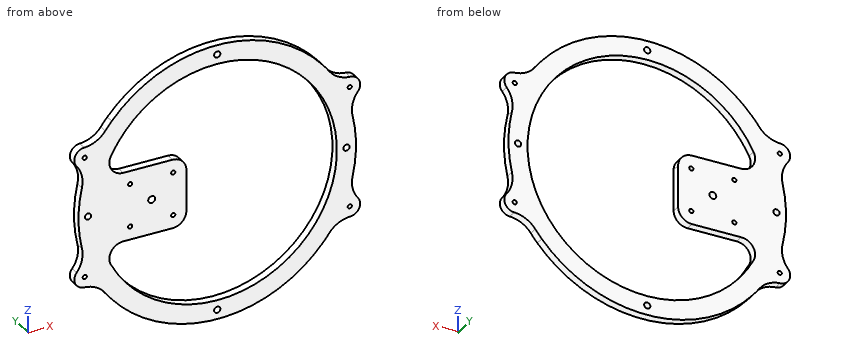
```python
from build123d import *

# Parameters (mm, degrees)
SKETCH1_R           = 86.25
BOSS_EXTRUDE1_DEPTH = 6
SKETCH2_R           = 1.5
CUT_EXTRUDE1_DEPTH  = 6
SKETCH3_R           = 2.25
CUT_EXTRUDE2_DEPTH  = 6
CUT_EXTRUDE3_DEPTH  = 6
FILLET1_R           = 20
SKETCH5_R           = 2.5
SKETCH5_R_2         = 1.5
BOSS_EXTRUDE2_DEPTH = 6
FILLET2_R           = 10


with BuildPart() as part:
    # Sketch1 → Boss-Extrude1 (new body)
    with BuildSketch(Plane(origin=(0, 0, 0), x_dir=(1, 0, 0), z_dir=(0, 1, 0))):
        with BuildLine():
            Line((75.993420768, 65), (110, 65))
            Line((110, 65), (110, -65))
            Line((110, -65), (75.993420768, -65))
            ThreePointArc((75.993420768, -65), (0, -100), (-75.993420768, -65))
            Line((-75.993420768, -65), (-110, -65))
            Line((-110, -65), (-110, 65))
            Line((-110, 65), (-75.993420768, 65))
            ThreePointArc((-75.993420768, 65), (0, 100), (75.993420768, 65))
        make_face()
        Circle(SKETCH1_R, mode=Mode.SUBTRACT)
    extrude(amount=BOSS_EXTRUDE1_DEPTH)

    # Sketch2 → Cut-Extrude1 (cut)
    with BuildSketch(Plane(origin=(0, 0, 0), x_dir=(1, 0, 0), z_dir=(0, 1, 0))):
        with Locations((-95.5, 43.5)):
            Circle(SKETCH2_R)
        with Locations((95.5, 43.5)):
            Circle(SKETCH2_R)
        with Locations((95.5, -43.5)):
            Circle(SKETCH2_R)
        with Locations((-95.5, -43.5)):
            Circle(SKETCH2_R)
    extrude(amount=CUT_EXTRUDE1_DEPTH, mode=Mode.SUBTRACT)

    # Sketch3 → Cut-Extrude2 (cut)
    with BuildSketch(Plane(origin=(0, 0, 0), x_dir=(1, 0, 0), z_dir=(0, 1, 0))):
        with Locations((0, 93.125)):
            Circle(SKETCH3_R)
        with Locations((93.125, 0)):
            Circle(SKETCH3_R)
        with Locations((0, -93.125)):
            Circle(SKETCH3_R)
        with Locations((-93.125, 0)):
            Circle(SKETCH3_R)
    extrude(amount=CUT_EXTRUDE2_DEPTH, mode=Mode.SUBTRACT)

    # Sketch4 → Cut-Extrude3 (cut)
    with BuildSketch(Plane(origin=(0, 0, 0), x_dir=(1, 0, 0), z_dir=(0, 1, 0))):
        with BuildLine():
            Line((98.608905775, -36.674701114), (93.856581268, -34.510029742))
            ThreePointArc((93.856581268, -34.510029742), (100, 0), (93.856581268, 34.510029742))
            Line((93.856581268, 34.510029742), (98.608905775, 36.674701114))
            ThreePointArc((98.608905775, 36.674701114), (102.325298886, 46.608905775), (92.391094225, 50.325298886))
            Line((92.391094225, 50.325298886), (87.638769717, 48.160627513))
            ThreePointArc((87.638769717, 48.160627513), (82.248188777, 56.879130117), (75.993420768, 65))
            Line((75.993420768, 65), (110, 65))
            Line((110, 65), (110, -65))
            Line((110, -65), (75.993420768, -65))
            ThreePointArc((75.993420768, -65), (82.248188777, -56.879130117), (87.638769717, -48.160627513))
            Line((87.638769717, -48.160627513), (92.391094225, -50.325298886))
            ThreePointArc((92.391094225, -50.325298886), (102.325298886, -46.608905775), (98.608905775, -36.674701114))
        make_face()
        with BuildLine():
            Line((-98.608905775, 36.674701114), (-93.856581268, 34.510029742))
            ThreePointArc((-93.856581268, 34.510029742), (-100, 0), (-93.856581268, -34.510029742))
            Line((-93.856581268, -34.510029742), (-98.608905775, -36.674701114))
            ThreePointArc((-98.608905775, -36.674701114), (-102.325298886, -46.608905775), (-92.391094225, -50.325298886))
            Line((-92.391094225, -50.325298886), (-87.638769717, -48.160627513))
            ThreePointArc((-87.638769717, -48.160627513), (-82.248188777, -56.879130117), (-75.993420768, -65))
            Line((-75.993420768, -65), (-110, -65))
            Line((-110, -65), (-110, 65))
            Line((-110, 65), (-75.993420768, 65))
            ThreePointArc((-75.993420768, 65), (-82.248188777, 56.879130117), (-87.638769717, 48.160627513))
            Line((-87.638769717, 48.160627513), (-92.391094225, 50.325298886))
            ThreePointArc((-92.391094225, 50.325298886), (-102.325298886, 46.608905775), (-98.608905775, 36.674701114))
        make_face()
    extrude(amount=CUT_EXTRUDE3_DEPTH, mode=Mode.SUBTRACT)

    # Fillet1
    fillet1_edges = [part.edges().sort_by_distance(p)[0] for p in [
        (87.638769717, 3, -48.160627513),
        (93.856581268, 3, -34.510029742),
        (93.856581268, 3, 34.510029742),
        (87.638769717, 3, 48.160627513),
        (-87.638769717, 3, 48.160627513),
        (-93.856581268, 3, 34.510029742),
        (-93.856581268, 3, -34.510029742),
        (-87.638769717, 3, -48.160627513),
    ]]
    fillet(fillet1_edges, radius=FILLET1_R)

    # Sketch5 → Boss-Extrude2 (add)
    with BuildSketch(Plane(origin=(0, 0, 0), x_dir=(1, 0, 0), z_dir=(0, 1, 0))):
        Polygon((-72.25, 25), (-22.25, 25), (-22.25, -25), (-72.25, -25), (-87.689436508, -25), (-87.689436508, 25), align=None)
        with Locations((-47.25, 0)):
            Circle(SKETCH5_R, mode=Mode.SUBTRACT)
        with Locations((-62.75, 15.5)):
            Circle(SKETCH5_R_2, mode=Mode.SUBTRACT)
        with Locations((-31.75, 15.5)):
            Circle(SKETCH5_R_2, mode=Mode.SUBTRACT)
        with Locations((-62.75, -15.5)):
            Circle(SKETCH5_R_2, mode=Mode.SUBTRACT)
        with Locations((-31.75, -15.5)):
            Circle(SKETCH5_R_2, mode=Mode.SUBTRACT)
    extrude(amount=BOSS_EXTRUDE2_DEPTH)

    # Fillet2
    fillet2_edges = [part.edges().sort_by_distance(p)[0] for p in [
        (-82.547334905, 3, 25),
        (-82.547334905, 3, -25),
        (-22.25, 3, 25),
        (-22.25, 3, -25),
    ]]
    fillet(fillet2_edges, radius=FILLET2_R)


solid = part.part
```
Can you work these out from the model? Positions are in its coordinate system, mm. Round coordinates to 2 decimals unless told otherwise and drop trailing zeros. Loops run counter-clockwise (first coordinate to the right, second up) from the corner with the lowest first, then second, coordinate; pieces in that order, holes last. Notation, with made-up numbers: M 21.5,63.5 L 61.5,63.5 A21 cw 61.5,92.5 Z; hole C 63,38 d8. An arc over 180 degrees is marked long. Answer as a JSON object with one key per item and string values. Group by question number.
Q1. Please list where these lines run through material, in increasing order: L1, parallel to Z at x = -95.5, y = 4.4; L2, parallel to Z at x = -47.25, y = 3.9; L3, parallel to Z at x = -54.5, y = 1.5.
Q2. Will these pins go through, and if not, where does the flat tip stop? pin 1 (3 mm diameter, centred on x = -41.5, y = 2.5, fed in from -Z); pin 2 (1.8 mm diameter, centred on x = -31.75, z = 15.5, fed in from +Y); pin 3 (1.5 mm diameter, centred on x = 55.5, y = 1, fed in from -Z); pin 4 (1.8 mm diameter, centred on y = 3, z = 2.5, fed in from +X).
Q3. Imagine slicing it at D-D, the plane y = 1.25. Count the separate pieces of the cut face and the enclosed holes in it, then the cut area to 3 significant figures.
Q4. Imagine slicing it at C-C, the plane z = -72. Please give me the cut outline in (x, y), then the cut area to 3 significant figures.
Q5. Imagine slicing it at A-A, the plane x = 27.5. Please give me the cut outline in (y, z), then the cut area to 3 significant figures.
Q6. Imagine slicing it at B-B, the plane x = -47.25. Please give me the cut outline in (y, z), then the cut area to 3 significant figures.
Findings:
{
 "1": {"L1": "z = -51.01 to -45, -42 to 42, 45 to 51.01", "L2": "z = -88.13 to -72.16, -25 to -2.5, 2.5 to 25, 72.16 to 88.13", "L3": "z = -83.84 to -66.85, -25 to 25, 66.85 to 83.84"},
 "2": {"pin 1": "stops at z = -91.65", "pin 2": "passes through", "pin 3": "stops at z = -83.68", "pin 4": "stops at x = 99.99"},
 "3": {"separate pieces": "1", "enclosed holes": "14", "area": "12,000 mm2"},
 "4": {"outline": "M -69.4,0 L -47.49,0 L -47.49,6 L -69.4,6 Z; M 47.49,0 L 69.4,0 L 69.4,6 L 47.49,6 Z", "area": "263 mm2"},
 "5": {"outline": "M 0,-96.14 L 6,-96.14 L 6,-81.75 L 0,-81.75 Z; M 0,81.75 L 6,81.75 L 6,96.14 L 0,96.14 Z", "area": "173 mm2"},
 "6": {"outline": "M 0,-88.13 L 6,-88.13 L 6,-72.16 L 0,-72.16 Z; M 0,-25 L 6,-25 L 6,-2.5 L 0,-2.5 Z; M 0,2.5 L 6,2.5 L 6,25 L 0,25 Z; M 0,72.16 L 6,72.16 L 6,88.13 L 0,88.13 Z", "area": "462 mm2"}
}
